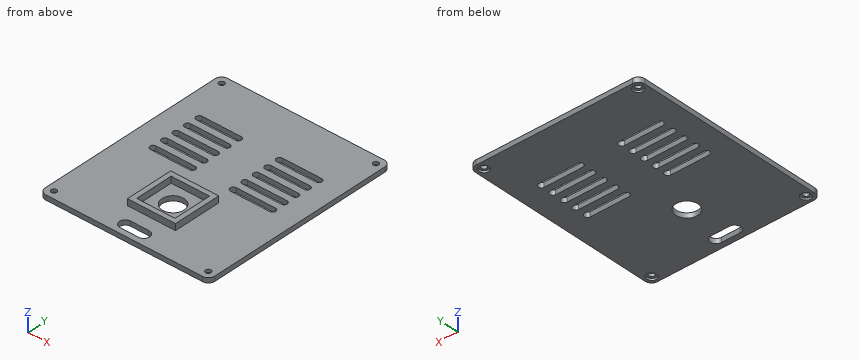
```python
from build123d import *

# Parameters (mm, degrees)
SKETCH_1_W          = 53
SKETCH_1_H          = 63
EXTRUDE_1_DEPTH     = 1.5
FILLET_1_R          = 2
CUT_EXTRUDE_2_DEPTH = 83.342273469
CUT_EXTRUDE_3_DEPTH = 83.342273469
SKETCH_5_R          = 3.45
CUT_EXTRUDE_4_DEPTH = 83.342273469
SKETCH_6_W          = 15
SKETCH_6_H          = 15
SKETCH_6_W_2        = 12
SKETCH_6_H_2        = 12
EXTRUDE_1_2_DEPTH   = 2
SKETCH_9_R          = 0.85
CUT_EXTRUDE_5_DEPTH = 83.402973247
SKETCH_10_R         = 1.55
CUT_EXTRUDE_6_DEPTH = 0.6


with BuildPart() as part:
    # 草图1 → Extrude 1 (new body)
    with BuildSketch(Plane.XY):
        with Locations((26.5, 31.5)):
            Rectangle(SKETCH_1_W, SKETCH_1_H)
    extrude(amount=EXTRUDE_1_DEPTH)

    # 圆角1
    fillet_1_edges = [part.edges().sort_by_distance(p)[0] for p in [
        (0, 63, 0.75),
        (53, 63, 0.75),
        (53, 0, 0.75),
        (0, 0, 0.75),
    ]]
    fillet(fillet_1_edges, radius=FILLET_1_R)

    # 草图3 → 切除-拉伸2 (cut, through all)
    with BuildSketch(Plane(origin=(0, 0, 0), x_dir=(-1, 0, 0), z_dir=(0, 0, -1))):
        with BuildLine():
            Line((-23.635661643, 5.35), (-29.435661643, 5.35))
            ThreePointArc((-29.435661643, 5.35), (-31.235661643, 3.55), (-29.435661643, 1.75))
            Line((-29.435661643, 1.75), (-23.635661643, 1.75))
            ThreePointArc((-23.635661643, 1.75), (-21.835661643, 3.55), (-23.635661643, 5.35))
        make_face()
    extrude(amount=-CUT_EXTRUDE_2_DEPTH, mode=Mode.SUBTRACT)

    # 草图4 → 切除-拉伸3 (cut, through all)
    with BuildSketch(Plane.XY.offset(1.5)):
        with BuildLine():
            Line((7.840284333, 47.730065189), (20.08572274, 47.730065189))
            ThreePointArc((20.08572274, 47.730065189), (21.057582931, 46.758204998), (20.08572274, 45.786344807))
            Line((20.08572274, 45.786344807), (7.840284333, 45.786344807))
            ThreePointArc((7.840284333, 45.786344807), (6.868424142, 46.758204998), (7.840284333, 47.730065189))
        make_face()
        with BuildLine():
            Line((7.840284333, 43.730065189), (20.08572274, 43.730065189))
            ThreePointArc((20.08572274, 43.730065189), (21.057582931, 42.758204998), (20.08572274, 41.786344807))
            Line((20.08572274, 41.786344807), (7.840284333, 41.786344807))
            ThreePointArc((7.840284333, 41.786344807), (6.868424142, 42.758204998), (7.840284333, 43.730065189))
        make_face()
        with BuildLine():
            Line((7.840284333, 39.730065189), (20.08572274, 39.730065189))
            ThreePointArc((20.08572274, 39.730065189), (21.057582931, 38.758204998), (20.08572274, 37.786344807))
            Line((20.08572274, 37.786344807), (7.840284333, 37.786344807))
            ThreePointArc((7.840284333, 37.786344807), (6.868424142, 38.758204998), (7.840284333, 39.730065189))
        make_face()
        with BuildLine():
            Line((7.840284333, 35.730065189), (20.08572274, 35.730065189))
            ThreePointArc((20.08572274, 35.730065189), (21.057582931, 34.758204998), (20.08572274, 33.786344807))
            Line((20.08572274, 33.786344807), (7.840284333, 33.786344807))
            ThreePointArc((7.840284333, 33.786344807), (6.868424142, 34.758204998), (7.840284333, 35.730065189))
        make_face()
        with BuildLine():
            Line((7.840284333, 31.730065189), (20.08572274, 31.730065189))
            ThreePointArc((20.08572274, 31.730065189), (21.057582931, 30.758204998), (20.08572274, 29.786344807))
            Line((20.08572274, 29.786344807), (7.840284333, 29.786344807))
            ThreePointArc((7.840284333, 29.786344807), (6.868424142, 30.758204998), (7.840284333, 31.730065189))
        make_face()
        with BuildLine():
            Line((45.159715667, 31.730065189), (32.91427726, 31.730065189))
            ThreePointArc((32.91427726, 31.730065189), (31.942417069, 30.758204998), (32.91427726, 29.786344807))
            Line((32.91427726, 29.786344807), (45.159715667, 29.786344807))
            ThreePointArc((45.159715667, 29.786344807), (46.131575858, 30.758204998), (45.159715667, 31.730065189))
        make_face()
        with BuildLine():
            Line((45.159715667, 35.730065189), (32.91427726, 35.730065189))
            ThreePointArc((32.91427726, 35.730065189), (31.942417069, 34.758204998), (32.91427726, 33.786344807))
            Line((32.91427726, 33.786344807), (45.159715667, 33.786344807))
            ThreePointArc((45.159715667, 33.786344807), (46.131575858, 34.758204998), (45.159715667, 35.730065189))
        make_face()
        with BuildLine():
            Line((45.159715667, 39.730065189), (32.91427726, 39.730065189))
            ThreePointArc((32.91427726, 39.730065189), (31.942417069, 38.758204998), (32.91427726, 37.786344807))
            Line((32.91427726, 37.786344807), (45.159715667, 37.786344807))
            ThreePointArc((45.159715667, 37.786344807), (46.131575858, 38.758204998), (45.159715667, 39.730065189))
        make_face()
        with BuildLine():
            Line((45.159715667, 43.730065189), (32.91427726, 43.730065189))
            ThreePointArc((32.91427726, 43.730065189), (31.942417069, 42.758204998), (32.91427726, 41.786344807))
            Line((32.91427726, 41.786344807), (45.159715667, 41.786344807))
            ThreePointArc((45.159715667, 41.786344807), (46.131575858, 42.758204998), (45.159715667, 43.730065189))
        make_face()
        with BuildLine():
            Line((45.159715667, 47.730065189), (32.91427726, 47.730065189))
            ThreePointArc((32.91427726, 47.730065189), (31.942417069, 46.758204998), (32.91427726, 45.786344807))
            Line((32.91427726, 45.786344807), (45.159715667, 45.786344807))
            ThreePointArc((45.159715667, 45.786344807), (46.131575858, 46.758204998), (45.159715667, 47.730065189))
        make_face()
    extrude(amount=-CUT_EXTRUDE_3_DEPTH, mode=Mode.SUBTRACT)

    # 草图5 → 切除-拉伸4 (cut, through all)
    with BuildSketch(Plane.XY.offset(1.5)):
        with Locations((26.5, 16.954492475)):
            Circle(SKETCH_5_R)
    extrude(amount=-CUT_EXTRUDE_4_DEPTH, mode=Mode.SUBTRACT)

    # 草图6 → Extrude 1 2 (add)
    with BuildSketch(Plane.XY.offset(1.5)):
        with Locations((26.5, 16.954492475)):
            Rectangle(SKETCH_6_W, SKETCH_6_H)
        with Locations((26.5, 16.954492475)):
            Rectangle(SKETCH_6_W_2, SKETCH_6_H_2, mode=Mode.SUBTRACT)
    extrude(amount=EXTRUDE_1_2_DEPTH)

    # 草图9 → 切除-拉伸5 (cut, through all)
    with BuildSketch(Plane(origin=(0, 0, 0), x_dir=(-1, 0, 0), z_dir=(0, 0, -1))):
        with Locations((-2.4, 2.4)):
            Circle(SKETCH_9_R)
        with Locations((-50.6, 60.6)):
            Circle(SKETCH_9_R)
        with Locations((-2.4, 60.6)):
            Circle(SKETCH_9_R)
        with Locations((-50.6, 2.4)):
            Circle(SKETCH_9_R)
    extrude(amount=-CUT_EXTRUDE_5_DEPTH, mode=Mode.SUBTRACT)

    # 草图10 → 切除-拉伸6 (cut)
    with BuildSketch(Plane(origin=(0, 0, 0), x_dir=(-1, 0, 0), z_dir=(0, 0, -1))):
        with Locations((-50.6, 60.6)):
            Circle(SKETCH_10_R)
        with Locations(Location((-2.4, 60.6, 0), (0, 0, 180))):
            Circle(SKETCH_10_R)
        with Locations((-2.4, 2.4)):
            Circle(SKETCH_10_R)
        with Locations(Location((-50.6, 2.4, 0), (0, 0, 180))):
            Circle(SKETCH_10_R)
    extrude(amount=-CUT_EXTRUDE_6_DEPTH, mode=Mode.SUBTRACT)


solid = part.part
```
Here's how the part is built. I have some questions about the finished solid (model axes, mm). Coordinates: 2 decimals unless noted, no trailing zeros. Order: outer loops, then holes, each group sorted by start corner. A loop starts at its lowest first (then second) coordinate and runs counter-clockwise, first axis right, second up. Notation, with made-up numbers: M 37.25,1.5 L 79.25,1.5 A22 cw 79.25,14.5 Z; hole C -8,61.5 d5. An arc over 180 degrees is marked long. Answer as a JSON object with one key per item and string values. Group by question number.
(1) For pin 1 (0.6 mm diameter, centred on y = 15, z = 3, fed in from +X); pin 2 (1.9 mm diameter, centred on x = 50.6, y = 60.6, fed in from +Z); pin 3 (10 mm diameter, centred on x = 24, y = 20.5, fed in from +Z); pin 4 (0.9 mm diameter, centred on x = 50, y = 60.5, fed in from -Z), each with a flat end and sliding along its axis, tell me the tip position at first contact or that it passes through.
(2) I need wall thicknesses on probe 1 along Y at (x, z) = (2.4, 0.4); probe 2 along X at (y, z) = (20, 2.45); probe 3 along Y at (x, z) = (42, 1.45). Which ranges of each line are inside material? Lowest first, please.
(3) Suppose I cut it at B-B, the plane y = 35. Please give me the cut outline in (x, z).
(4) Suppose I cut it at D-D, the plane x = 11. Please give me the cut outline in (y, z).
(5) Suppose I cut it at A-A, the plane z = 2.5. Please give me the cut outline in (x, y).
(6) Suppose I cut it at C-C, the plane x = 26.5. Please give me the cut outline in (y, z).
Values found:
{
 "1": {"pin 1": "stops at x = 34", "pin 2": "stops at z = 1.5", "pin 3": "stops at z = 3.5", "pin 4": "stops at z = 0.6"},
 "2": {"probe 1": "y = 0 to 0.85, 3.95 to 59.05, 62.15 to 63", "probe 2": "x = 19 to 20.5, 32.5 to 34", "probe 3": "y = 0 to 29.79, 31.73 to 33.79, 35.73 to 37.79, 39.73 to 41.79, 43.73 to 45.79, 47.73 to 63"},
 "3": {"outline": "M 0,0 L 6.9,0 L 6.9,1.5 L 0,1.5 Z; M 21.03,0 L 31.97,0 L 31.97,1.5 L 21.03,1.5 Z; M 46.1,0 L 53,0 L 53,1.5 L 46.1,1.5 Z"},
 "4": {"outline": "M 0,0 L 29.79,0 L 29.79,1.5 L 0,1.5 Z; M 31.73,0 L 33.79,0 L 33.79,1.5 L 31.73,1.5 Z; M 35.73,0 L 37.79,0 L 37.79,1.5 L 35.73,1.5 Z; M 39.73,0 L 41.79,0 L 41.79,1.5 L 39.73,1.5 Z; M 43.73,0 L 45.79,0 L 45.79,1.5 L 43.73,1.5 Z; M 47.73,0 L 63,0 L 63,1.5 L 47.73,1.5 Z"},
 "5": {"outline": "M 19,9.45 L 34,9.45 L 34,24.45 L 19,24.45 Z; hole M 20.5,10.95 L 32.5,10.95 L 32.5,22.95 L 20.5,22.95 Z"},
 "6": {"outline": "M 0,0 L 1.75,0 L 1.75,1.5 L 0,1.5 Z; M 5.35,0 L 13.5,0 L 13.5,1.5 L 10.95,1.5 L 10.95,3.5 L 9.45,3.5 L 9.45,1.5 L 5.35,1.5 Z; M 20.4,0 L 63,0 L 63,1.5 L 24.45,1.5 L 24.45,3.5 L 22.95,3.5 L 22.95,1.5 L 20.4,1.5 Z"}
}
